```python
from build123d import *

# Parameters (mm, degrees)
SKETCH2_R               = 13.5
BOSS_EXTRUDE1_DEPTH     = 6
SKETCH3_R               = 6.5
SKETCH3_R_2             = 2.5
BOSS_EXTRUDE2_DEPTH     = 10
SKETCH4_R               = 1.2
CUT_EXTRUDE1_DEPTH      = 25
CUT_EXTRUDE1_DEPTH_BACK = 25
SKETCH6_R               = 2.7
CUT_EXTRUDE3_DEPTH      = 50
CUT_EXTRUDE3_DEPTH_BACK = 20
SKETCH5_R               = 2.3
CUT_EXTRUDE4_DEPTH      = 10
SKETCH8_W               = 10
SKETCH8_H               = 1
CUT_EXTRUDE5_DEPTH      = 1


with BuildPart() as part:
    # Sketch2 → Boss-Extrude1 (new body)
    with BuildSketch(Plane.XY):
        Circle(SKETCH2_R)
    extrude(amount=BOSS_EXTRUDE1_DEPTH)

    # Sketch3 → Boss-Extrude2 (add)
    with BuildSketch(Plane.XY.offset(6)):
        Circle(SKETCH3_R)
        Circle(SKETCH3_R_2, mode=Mode.SUBTRACT)
    extrude(amount=BOSS_EXTRUDE2_DEPTH)

    # Sketch4 → Cut-Extrude1 (cut, two sides)
    with BuildSketch(Plane(origin=(0, 0, 0), x_dir=(0, -1, 0), z_dir=(1, 0, 0))) as cut_extrude1_sk:
        with Locations((0, -11)):
            Circle(SKETCH4_R)
    extrude(amount=CUT_EXTRUDE1_DEPTH, mode=Mode.SUBTRACT)
    extrude(cut_extrude1_sk.sketch, amount=-CUT_EXTRUDE1_DEPTH_BACK, mode=Mode.SUBTRACT)

    # Sketch6 → Cut-Extrude3 (cut, two sides)
    with BuildSketch(Plane.XY.offset(6)) as cut_extrude3_sk:
        Circle(SKETCH6_R)
    extrude(amount=CUT_EXTRUDE3_DEPTH, mode=Mode.SUBTRACT)
    extrude(cut_extrude3_sk.sketch, amount=-CUT_EXTRUDE3_DEPTH_BACK, mode=Mode.SUBTRACT)

    # Sketch5 → Cut-Extrude4 (cut)
    with BuildSketch(Plane.XY.offset(6)):
        with Locations((0, 10)):
            Circle(SKETCH5_R)
    cut_extrude4 = extrude(amount=-CUT_EXTRUDE4_DEPTH, mode=Mode.SUBTRACT)

    # Mirror1: Cut-Extrude4 across plane
    add(cut_extrude4.mirror(Plane.ZX), mode=Mode.SUBTRACT)

    # Sketch8 → Cut-Extrude5 (cut)
    with BuildSketch(Plane(origin=(0, 0, 0), x_dir=(-1, 0, 0), z_dir=(0, 0, -1))):
        with Locations((-13.5, 0)):
            Rectangle(SKETCH8_W, SKETCH8_H)
    cut_extrude5 = extrude(amount=-CUT_EXTRUDE5_DEPTH, mode=Mode.SUBTRACT)

    # Mirror2: Cut-Extrude5 across plane
    add(cut_extrude5.mirror(Plane(origin=(0, 0, 0), x_dir=(0, 0, 1), z_dir=(1, 0, 0))), mode=Mode.SUBTRACT)


solid = part.part
```
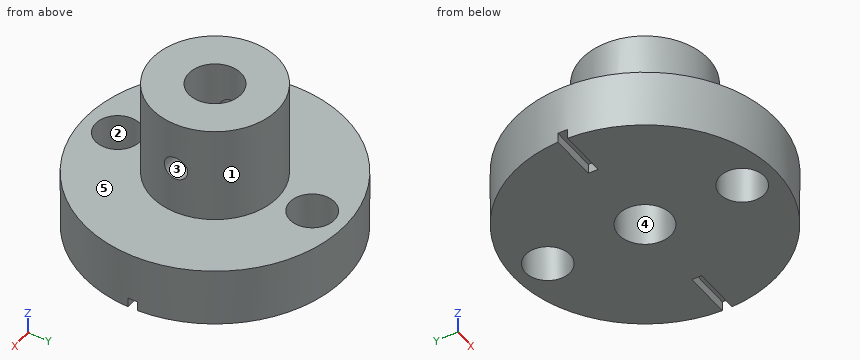
Could you check a few things on this model? Use its own coordinates, in mm. Face numbers are marked on the shaded views. A direction names the side the tool comes from. Give positions to 0.01 mm unless a question says otherwise; leave off trailing zeros. Loops run counter-clockwise (first coordinate to the right, second up) from the corner with the lowest first, then second, coordinate; pieces in that order, holes last. Notation, with made-up numbers: (-25.75, -17) - (6.25, -17) arc R15 ccw to (6.25, -3) - close; hole circle Ø4 at (10, 76.25). An arc over 180 degrees is marked (long way). Answer in a Markdown table with one row per item. Add a question column.
Q1. Please list where these lines run through material, in increasing order: L1, parallel to Y at x = 0, z = 2.5; L2, parallel to Y at x = 0, z = 10.5. Write a range as from..to.
Q2. If we section it at A-A (y = 0): List the corners of the cut face in (x, z) for me, plus the area to 3 significant figures.
Q3. For pin 1 (3 mm diameter, centred on x = -4, z = 9.5, fed in from -Y); pin 2 (3 mm diameter, centred on x = 0, y = 10, fed in from -Z); pin 3 (0.8 mm diameter, centred on x = -12, y = 0, fed in from -Z); pin 4 (1 mm diameter, centred on x = 4.5, z = 3, fed in from +Y), each with a flat end and sliding along its axis, tell me the tip position at first contact or that it passes through.
Q4. If we section it at D-D (x = -1.5): List the corners of the cut face in (y, z) for me (3 decimals).
Q5. If we section it at C-C (y = -11): List the corners of the cut face in (x, z) for me.
Q6. We'd pull the mould along X, two halves only. Please class the marked faces 1, 2 and 3: +X half, -X half, draft (parallel to the pull), parting line (faces both ways), or undercut.
Q7. If we section it at B-B (z = 11): List the corners of the cut face in (x, y) for me, plus the area to 3 significant figures.
Q8. Which directions (+Z, -Z, +X, -X, +Y, -Y) give clear straight access to the entire face, cutting with the end or side of a thin tool? Please do the marked faces 4 and 5.
The answers:
| question | item | result |
|---|---|---|
| 1 | L1 | y = -13.5..-12.3, -7.7..-2.7, 2.7..7.7, 12.3..13.5 |
| 1 | L2 | y = -6.5..-2.7, 2.7..6.5 |
| 2 | outline | (-13.5, 1) - (-8.5, 1) - (-8.5, 0) - (-2.7, 0) - (-2.7, 9.8) - (-6.5, 9.8) - (-6.5, 6) - (-13.5, 6) - close; (-6.5, 12.2) - (-2.7, 12.2) - (-2.7, 16) - (-6.5, 16) - close; (2.7, 0) - (8.5, 0) - (8.5, 1) - (13.5, 1) - (13.5, 6) - (6.5, 6) - (6.5, 9.8) - (2.7, 9.8) - close; (2.7, 12.2) - (6.5, 12.2) - (6.5, 16) - (2.7, 16) - close |
| 2 | area | 177 mm^2 |
| 3 | pin 1 | stops at y = -6 |
| 3 | pin 2 | passes through |
| 3 | pin 3 | stops at z = 1 |
| 3 | pin 4 | stops at y = 12.89 |
| 4 | outline | (-13.416, 0) - (-11.744, 0) - (-11.744, 6) - (-13.416, 6) - close; (-8.256, 0) - (-2.245, 0) - (-2.245, 16) - (-6.325, 16) - (-6.325, 6) - (-8.256, 6) - close; (2.245, 0) - (8.256, 0) - (8.256, 6) - (6.325, 6) - (6.325, 16) - (2.245, 16) - close; (11.744, 0) - (13.416, 0) - (13.416, 6) - (11.744, 6) - close |
| 5 | outline | (-7.83, 0) - (-2.07, 0) - (-2.07, 6) - (-7.83, 6) - close; (2.07, 0) - (7.83, 0) - (7.83, 6) - (2.07, 6) - close |
| 6 | face 1 | parting line |
| 6 | face 2 | undercut |
| 6 | face 3 | draft |
| 7 | outline | (-6.39, -1.2) arc R6.5 ccw to (6.39, -1.2) - (2.42, -1.2) arc R2.7 cw to (-2.42, -1.2) - close; (-6.39, 1.2) - (-2.42, 1.2) arc R2.7 cw to (2.42, 1.2) - (6.39, 1.2) arc R6.5 ccw to start |
| 7 | area | 91.3 mm^2 |
| 8 | face 4 | +Z, -Z |
| 8 | face 5 | +Z |
